```python
from build123d import *

# Parameters (mm, degrees)
EXTRUDE_1_DEPTH     = 20
FILLET_1_R          = 3
FILLET_2_R          = 3
SKETCH_3_R          = 2.1
CUT_EXTRUDE_1_DEPTH = 10


with BuildPart() as part:
    # 草图1 → 凸台-拉伸1 (new body)
    with BuildSketch(Plane(origin=(0, 0, 0), x_dir=(1, 0, 0), z_dir=(0, 1, 0))):
        Polygon((-21.2, 6.013269655), (-21.2, 0), (-41.2, 0), (-41.2, 3), (-24.2, 3), (-24.2, 45.2), (24.2, 45.2), (24.2, 3), (41.2, 3), (41.2, 0), (21.2, 0), (21.2, 6.013269655), (21.2, 42.2), (-21.2, 42.2), align=None)
    extrude(amount=EXTRUDE_1_DEPTH)

    # 圆角1
    fillet_1_edges = [part.edges().sort_by_distance(p)[0] for p in [
        (-24.2, 10, -45.2),
        (24.2, 10, -45.2),
    ]]
    fillet(fillet_1_edges, radius=FILLET_1_R)

    # 圆角2
    fillet_2_edges = [part.edges().sort_by_distance(p)[0] for p in [
        (-41.2, 20, -1.5),
        (41.2, 0, -1.5),
        (-41.2, 0, -1.5),
        (41.2, 20, -1.5),
    ]]
    fillet(fillet_2_edges, radius=FILLET_2_R)

    # 草图3 → 切除-拉伸1 (cut)
    with BuildSketch(Plane(origin=(0, 0, -3), x_dir=(-1, 0, 0), z_dir=(0, 0, -1))):
        with Locations((31.2, 10)):
            Circle(SKETCH_3_R)
        with Locations((-31.2, 10)):
            Circle(SKETCH_3_R)
    extrude(amount=-CUT_EXTRUDE_1_DEPTH, mode=Mode.SUBTRACT)


solid = part.part
```
Source: CAD feature listing. Evaluate the final solid. Frame: model axes, mm. A direction names the side the tool comes from. Give positions to 0.01 mm unless a question says otherwise; leave off trailing zeros. Write each loop counter-clockwise with the first axis right and the second up, starting at its lowest first coordinate (ties: lowest second). Pieces come first, ordered by that corner, then holes.
1. Material intervals for line 1 along Y through (x, z) = (31.2, -2); line 2 along X through (y, z) = (1, -29.5); line 3 along Z through (x, y) = (12, 16), sorted ascending.
2. First-contact query: pin 1 (4 mm diameter, centred on y = 9.5, z = -34, fed in from +X); pin 2 (12 mm diameter, centred on x = -3.5, y = 15.5, fed in from +Z); pin 3 (10 mm diameter, centred on y = 14.5, z = -18.5, fed in from -X). Flat tips, straight axial feed; report the tip coordinate or a pass-through.
3. Section query B-B (x = 31.2). Return the cut outline in (y, z).
4. Access query for faces 1 (the face through (34, 10, -3)), 2 (the face through (-35, 10, -3)), 3 (the face through (21.2, 10, -21)), 4 (the face through (-29.1, 10.09, -1.52)). Directions: +Z, -Z, +X, -X, +Y, -Y. A direction counts if a zero-diameter tool reaches every point of the face in a straight line with its end or side. Return the directions, or none.
5. Pull-direction query (X, two-part tool) for faces 5 (the face through (31.473, 12.082, -1.521)), 6 (the face through (41.2, 10, -2)), 7 (the face through (31.3, 7.6, 0)); classes: +X half, -X half, draft (parallel to the pull), parting line (faces both ways), or undercut.
6. Section query A-A (y = 10). Return the cut outline in (x, z), then the cut area to 3 significant figures.
7. Section query C-C (z = -40.5). Return the cut outline in (x, y).
8. Section query D-D (y = 15). Return the cut outline in (x, z), then the cut area to 3 significant figures.
Output values:
1. line 1: y = 0 to 7.9, 12.1 to 20
1. line 2: x = -24.2 to -21.2, 21.2 to 24.2
1. line 3: z = -45.2 to -42.2
2. pin 1: stops at x = 24.2
2. pin 2: stops at z = -42.2
2. pin 3: stops at x = -24.2
3. outline: (0, -3) - (7.9, -3) - (7.9, 0) - (0, 0) - close; (12.1, -3) - (20, -3) - (20, 0) - (12.1, 0) - close
4. face 1: -Z, +X, +Y, -Y
4. face 2: -Z, -X, +Y, -Y
4. face 3: +Z, +Y, -Y
4. face 4: +Z, -Z
5. face 5: undercut
5. face 6: +X half
5. face 7: draft
6. outline: (-41.2, -3) - (-33.3, -3) - (-33.3, 0) - (-41.2, 0) - close; (-29.1, -3) - (-24.2, -3) - (-24.2, -42.2) arc R3 ccw to (-21.2, -45.2) - (21.2, -45.2) arc R3 ccw to (24.2, -42.2) - (24.2, -3) - (29.1, -3) - (29.1, 0) - (21.2, 0) - (21.2, -42.2) - (-21.2, -42.2) - (-21.2, 0) - (-29.1, 0) - close; (33.3, -3) - (41.2, -3) - (41.2, 0) - (33.3, 0) - close
6. area: 471 mm2
7. outline: (-24.2, 0) - (-21.2, 0) - (-21.2, 20) - (-24.2, 20) - close; (21.2, 0) - (24.2, 0) - (24.2, 20) - (21.2, 20) - close
8. outline: (-41.2, -3) - (-24.2, -3) - (-24.2, -42.2) arc R3 ccw to (-21.2, -45.2) - (21.2, -45.2) arc R3 ccw to (24.2, -42.2) - (24.2, -3) - (41.2, -3) - (41.2, 0) - (21.2, 0) - (21.2, -42.2) - (-21.2, -42.2) - (-21.2, 0) - (-41.2, 0) - close
8. area: 497 mm2
